CAD build for the part. Positions are in the model's coordinates, mm. Face numbers are marked on the shaded views. A direction names the side the tool comes from. Give positions to 0.01 mm unless a question says otherwise; leave off trailing zeros. Order: outer loops, then holes, each group sorted by start corner. A loop starts at its lowest first (then second) coordinate and runs counter-clockwise, first axis right, second up. Notation, with made-up numbers: M 89,-38.5 L 141,-38.5 A21 ccw 141,-26.5 Z; hole C -27,-7.75 d6. An arc over 180 degrees is marked long. Put each result on its own line as item: value. Start each with the question number.
1) Drill centre lines: line 1 (Y direction, x = 9, z = 18.5); line 2 (Z direction, x = -12, y = 11); line 3 (X direction, y = 24, z = 20.5). Where is each one in solid material? Low to high. Write a range as [from, to].
2) Pin check, flat tips, straight feed: pin 1 (10 mm diameter, centred on y = 0.5, z = 14, fed in from -X); pin 2 (5.5 mm diameter, centred on x = -13, y = 24.5, fed in from -Z); pin 3 (3 mm diameter, centred on y = 18, z = 18, fed in from +X); pin 4 (10 mm diameter, centred on y = 4.5, z = 5.5, fed in from +X). Stop position of each tip, or through.
3) Cut at C-C (z = 22.25). Write the cut outline in (x, y).
4) Cut at D-D (y = 10). Write the cut outline in (x, z).
5) Tool access for the marked faces 5, 6, 7 and 8: list every direction of +Z, -Z, +X, -X, +Y, -Y with a clear straight run to the whole face (end or side of a thin tool).
6) Two-plate mould, pull along Y, no slides. Class the marked faces 1, 2, 3 and 4: released by +Y, released by -Y, zero draft, split by the parting line, or undercut.
7) Cut at B-B (x = 2). Write the cut outline in (y, z), and give its area (3 significant figures).
8) Cut at A-A (z = 17.25). Write the cut outline in (x, y).
```python
from build123d import *

# Parameters (mm, degrees)
F1_DEPTH       = 25.4
F2_DEPTH       = 15.24
F3_D           = 3.4544
F3_START       = 15.24
F3_CSINK_D     = 9.1186
F3_CSINK_ANGLE = 82
F4_R           = 5.08
F5_SIZE        = 10.16


with BuildPart() as f1:
    # F0 (on Top) → F1 (new body)
    with BuildSketch(Plane.XY):
        Polygon((-7.5087412455, 6.2847674176), (-19.9657089517, 6.2847674176), (-19.9657089517, -6.4152325824), (18.1342910483, -6.4152325824), (18.1342910483, 6.2847674176), align=None)
        with BuildLine():
            Line((-20.1363313266, 25.3347674176), (-19.9657089517, 6.2847674176))
            Line((-19.9657089517, 6.2847674176), (-7.5087412455, 6.2847674176))
            Line((-7.5087412455, 6.2847674176), (-7.5087412455, 25.3347674176))
            ThreePointArc((-7.5087412455, 25.3347674176), (-13.8225362861, 32.3618879282), (-20.1363313266, 25.3347674176))
        make_face()
    extrude(amount=F1_DEPTH)

    # F0 (on Top) → F2 (cut)
    with BuildSketch(Plane.XY):
        with BuildLine():
            Line((-20.1363313266, 25.3347674176), (-19.9657089517, 6.2847674176))
            Line((-19.9657089517, 6.2847674176), (-7.5087412455, 6.2847674176))
            Line((-7.5087412455, 6.2847674176), (-7.5087412455, 25.3347674176))
            ThreePointArc((-7.5087412455, 25.3347674176), (-13.8225362861, 32.3618879282), (-20.1363313266, 25.3347674176))
        make_face()
    extrude(amount=F2_DEPTH, mode=Mode.SUBTRACT)

    # F3 (through all)
    # its depths count from where the whole tool has entered the part; down to there all is cleared
    with Locations(Plane(origin=(0, 0, 0), x_dir=(1, 0, 0), z_dir=(0, 0, -1)).offset(-F3_START)):
        with Locations((-13.8225362861, -26.0118879282)):
            CounterSinkHole(F3_D / 2, F3_CSINK_D / 2, counter_sink_angle=F3_CSINK_ANGLE)

    # F4
    f4_edges = [f1.edges().sort_by_distance(p)[0] for p in [
        (-7.508741, 6.284767, 20.32),
    ]]
    fillet(f4_edges, radius=F4_R)

    # F5
    f5_edges = [f1.edges().sort_by_distance(p)[0] for p in [
        (18.134291, -0.065233, 0),
    ]]
    chamfer(f5_edges, length=F5_SIZE)


solid = f1.part
```
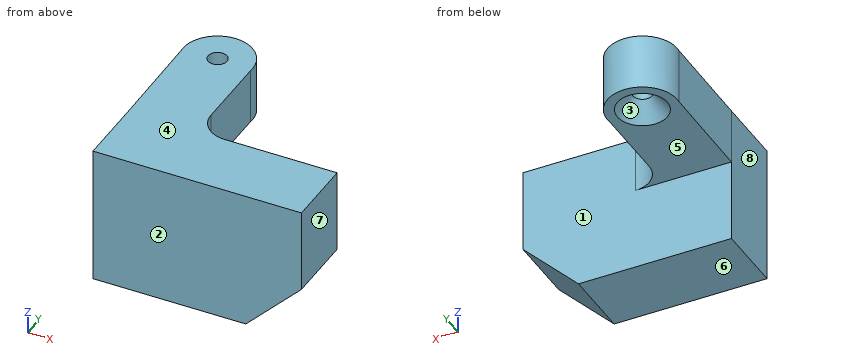
Solution:
1. line 1: [-6.42, 6.28]
1. line 2: [15.24, 25.4]
1. line 3: [-20.12, -7.51]
2. pin 1: x = -19.97
2. pin 2: z = 15.34
2. pin 3: x = -7.51
2. pin 4: x = 18.13
3. outline: M -20.14,25.33 L -19.97,6.28 L -19.97,-6.42 L 18.13,-6.42 L 18.13,6.28 L -2.43,6.28 A5.08 cw -7.51,11.36 L -7.51,25.33 A6.35 ccw long Z; hole C -13.82,26.01 d3.45
4. outline: M -20,15.24 L -7.32,15.24 L -7.32,25.4 L -20,25.4 Z
5. face 5: -Z, +X, -X, +Y
5. face 6: -Z, +X, -X, +Y, -Y
5. face 7: +Z, -Z, +X, +Y, -Y
5. face 8: +Z, -Z, -X, -Y
6. face 1: released by +Y
6. face 2: released by -Y
6. face 3: undercut
6. face 4: zero draft
7. outline: M -6.42,0 L 6.28,0 L 6.28,25.4 L -6.42,25.4 Z
7. area: 323 mm²
8. outline: M -20.14,25.33 L -19.97,6.28 L -19.97,-6.42 L 18.13,-6.42 L 18.13,6.28 L -2.43,6.28 A5.08 cw -7.51,11.36 L -7.51,25.33 A6.35 ccw long Z; hole C -13.82,26.01 d5.62
